from build123d import *

# Parameters (mm, degrees)
F0_R     = 11.05
F1_DEPTH = 3.5
F2_DEPTH = 2.5


with BuildPart() as f1:
    # F0 (on Top) → F1 (new body, symmetric)
    with BuildSketch(Plane.XY):
        with BuildLine():
            Line((16.4067340595, 45.3467654298), (8.4209065052, 43.9228967168))
            ThreePointArc((8.4209065052, 43.9228967168), (15.6672457553, 43.3028857057), (21.6327540042, 39.1427706216))
            Line((21.6327540042, 39.1427706216), (16.4067340595, 45.3467654298))
        make_face()
        with BuildLine():
            Line((0.4350802259, 42.4990282311), (-2.3247269809, 34.8711645999))
            ThreePointArc((-2.3247269809, 34.8711645999), (1.8353876304, 40.8366725376), (8.4209065052, 43.9228967168))
            Line((8.4209065052, 43.9228967168), (0.4350802259, 42.4990282311))
        make_face()
        with BuildLine():
            ThreePointArc((24.9371199001, 30.0910388701), (24.7259953173, 27.6645131258), (24.0989665638, 25.3109125396))
            Line((24.0989665638, 25.3109125396), (26.8587737337, 32.9387760688))
            Line((26.8587737337, 32.9387760688), (21.6327540042, 39.1427706216))
            ThreePointArc((21.6327540042, 39.1427706216), (24.0852004265, 34.9090436873), (24.9371199001, 30.0910388701))
        make_face()
        with BuildLine():
            Line((-5.0845339335, 27.2433016714), (-0.112226606, 21.3404981668))
            Line((-0.112226606, 21.3404981668), (-0.1100221461, 21.3465910994))
            ThreePointArc((-0.1100221461, 21.3465910994), (-2.9782076587, 27.8205341493), (-2.3247269809, 34.8711645999))
            Line((-2.3247269809, 34.8711645999), (-5.0845339335, 27.2433016714))
        make_face()
        with BuildLine():
            Line((13.7432325819, 16.334399733), (13.741028122, 16.3283068004))
            Line((13.741028122, 16.3283068004), (21.3391595743, 17.6830495091))
            Line((21.3391595743, 17.6830495091), (24.0989665638, 25.3109125396))
            ThreePointArc((24.0989665638, 25.3109125396), (20.0897974955, 19.474390384), (13.7432325819, 16.334399733))
        make_face()
        with BuildLine():
            Line((-0.112226606, 21.3404981668), (0.1414857049, 21.0393072268))
            ThreePointArc((0.1414857049, 21.0393072268), (0.0146461468, 21.1920605869), (-0.1100221461, 21.3465910994))
            Line((-0.1100221461, 21.3465910994), (-0.112226606, 21.3404981668))
        make_face()
        with BuildLine():
            ThreePointArc((13.7432325819, 16.334399733), (13.5485483413, 16.2954128005), (13.3533326046, 16.2591809003))
            Line((13.3533326046, 16.2591809003), (13.741028122, 16.3283068004))
            Line((13.741028122, 16.3283068004), (13.7432325819, 16.334399733))
        make_face()
        Polygon((18.5375268448, -10.5730579916), (11.3795390219, -11.8493233304), (10.9594646934, -13.0103717128), (9.743930135, -13.227100864), (7.2702144289, -20.064232828), (4.6443903041, -27.3217790413), (15.0964299783, -39.7297684023), (31.0680838119, -36.8820312036), (36.5876979713, -21.6263046439), (26.1356582971, -9.2183152829), align=None)
        with Locations((20.6160441377, -24.4740418426)):
            Circle(F0_R, mode=Mode.SUBTRACT)
        Polygon((-16.7470447626, -2.98598898), (-16.3269704341, -1.8249405976), (-21.0112425509, 3.7359260276), (-25.9835498784, 9.6387295322), (-41.955203712, 6.7909923335), (-47.4748178714, -8.4647342262), (-37.0227781972, -20.8727235872), (-21.0511243636, -18.0249863885), (-18.4253002388, -10.7674401752), (-15.9515845328, -3.9303082112), align=None)
        with Locations((-31.5031640378, -5.6169970275)):
            Circle(F0_R, mode=Mode.SUBTRACT)
        with BuildLine():
            ThreePointArc((0.1414857049, 21.0393072268), (2.850394978, 18.5665626335), (6.106993819, 16.8791921162))
            ThreePointArc((6.106993819, 16.8791921162), (9.6893501995, 16.092187212), (13.3533326046, 16.2591809003))
            ThreePointArc((13.3533326046, 16.2591809003), (13.5485483413, 16.2954128005), (13.7432325819, 16.334399733))
            ThreePointArc((13.7432325819, 16.334399733), (20.0897974955, 19.474390384), (24.0989665638, 25.3109125396))
            ThreePointArc((24.0989665638, 25.3109125396), (24.7259953173, 27.6645131258), (24.9371199001, 30.0910388701))
            ThreePointArc((24.9371199001, 30.0910388701), (24.0852004265, 34.9090436873), (21.6327540042, 39.1427706216))
            ThreePointArc((21.6327540042, 39.1427706216), (15.6672457553, 43.3028857057), (8.4209065052, 43.9228967168))
            ThreePointArc((8.4209065052, 43.9228967168), (1.8353876304, 40.8366725376), (-2.3247269809, 34.8711645999))
            ThreePointArc((-2.3247269809, 34.8711645999), (-2.9782076587, 27.8205341493), (-0.1100221461, 21.3465910994))
            ThreePointArc((-0.1100221461, 21.3465910994), (0.0146461468, 21.1920605869), (0.1414857049, 21.0393072268))
        make_face()
        with BuildLine():
            ThreePointArc((21.9371199001, 30.0910388701), (17.2337915702, 21.0454731767), (7.1276613096, 19.7002270103))
            ThreePointArc((7.1276613096, 19.7002270103), (4.5404482301, 39.1366045634), (21.9371199001, 30.0910388701))
        make_face(mode=Mode.SUBTRACT)
        Polygon((6.5830402991, 15.0520414616), (5.3675057407, 14.8353123104), (4.5720455108, 15.7796315416), (-2.5859423121, 14.5033662028), (-10.9594646934, 13.0103717128), (-13.853254728, 5.0121913664), (-16.3269704341, -1.8249405976), (-15.5315102042, -2.7692598288), (-15.9515845328, -3.9303082112), (-11.2673124159, -9.4911748364), (-5.7875800692, -15.9963606927), (2.5859423121, -14.5033662028), (9.743930135, -13.227100864), (10.1640044635, -12.0660524816), (11.3795390219, -11.8493233304), (13.853254728, -5.0121913664), (16.7470447626, 2.98598898), (11.2673124159, 9.4911748364), align=None)
        with BuildLine():
            ThreePointArc((3.7594585905, 10.3908118598), (9.0455656933, 6.3466716701), (11.05, 0))
            ThreePointArc((11.05, 0), (-9.0455656933, -6.3466716701), (3.7594585905, 10.3908118598))
        make_face(mode=Mode.SUBTRACT)
        with BuildLine():
            Line((6.106993819, 16.8791921162), (5.7875800692, 15.9963606927))
            Line((5.7875800692, 15.9963606927), (6.5830402991, 15.0520414616))
            Line((6.5830402991, 15.0520414616), (13.3533326046, 16.2591809003))
            ThreePointArc((13.3533326046, 16.2591809003), (9.6893501995, 16.092187212), (6.106993819, 16.8791921162))
        make_face()
        with BuildLine():
            Line((4.5720455108, 15.7796315416), (5.7875800692, 15.9963606927))
            Line((5.7875800692, 15.9963606927), (6.106993819, 16.8791921162))
            ThreePointArc((6.106993819, 16.8791921162), (2.850394978, 18.5665626335), (0.1414857049, 21.0393072268))
            Line((0.1414857049, 21.0393072268), (4.5720455108, 15.7796315416))
        make_face()
        Polygon((4.5720455108, 15.7796315416), (5.3675057407, 14.8353123104), (5.7875800692, 15.9963606927), align=None)
        Polygon((5.7875800692, 15.9963606927), (5.3675057407, 14.8353123104), (6.5830402991, 15.0520414616), align=None)
        Polygon((10.9594646934, -13.0103717128), (11.3795390219, -11.8493233304), (10.1640044635, -12.0660524816), (9.743930135, -13.227100864), align=None)
        Polygon((-15.5315102042, -2.7692598288), (-16.3269704341, -1.8249405976), (-16.7470447626, -2.98598898), (-15.9515845328, -3.9303082112), align=None)
    extrude(amount=F1_DEPTH, both=True)

    # F0 (on Top) → F2 (join, symmetric)
    with BuildSketch(Plane.XY):
        Polygon((-2.5859423121, 14.5033662028), (4.5720455108, 15.7796315416), (0.1414857049, 21.0393072268), (-0.112226606, 21.3404981668), align=None)
        Polygon((13.3533326046, 16.2591809003), (6.5830402991, 15.0520414616), (11.2673124159, 9.4911748364), (13.741028122, 16.3283068004), align=None)
        Polygon((18.5375268448, -10.5730579916), (13.853254728, -5.0121913664), (11.3795390219, -11.8493233304), align=None)
        Polygon((7.2702144289, -20.064232828), (9.743930135, -13.227100864), (2.5859423121, -14.5033662028), align=None)
        Polygon((-11.2673124159, -9.4911748364), (-15.9515845328, -3.9303082112), (-18.4253002388, -10.7674401752), align=None)
        Polygon((-16.3269704341, -1.8249405976), (-13.853254728, 5.0121913664), (-21.0112425509, 3.7359260276), align=None)
    extrude(amount=F2_DEPTH, both=True)


solid = f1.part
For this review, take the finished solid that the model builds, in its own axes (mm). A direction names the side the tool comes from. Give positions to 0.01 mm unless a question says otherwise; leave off trailing zeros. Loops run counter-clockwise (first coordinate to the right, second up) from the corner with the lowest first, then second, coordinate; pieces in that order, holes last.
Item 1: For line 1 along X through (y, z) = (-13, -0.5); line 2 along X through (y, z) = (40, 0.5); line 3 along Y through (x, z) = (-30.5, -2.25), list the stretches that pass through material, from the lowest coordinate up.
Item 2: Tool access review of faces 4 (the flat face through (-15, -8, 2.5)), 5 (the flat face through (4.895, -17.245, -0.035)), 6 (the flat face through (7, -16, -2.5)): name each direction out of +Z, -Z, +X, -X, +Y, -Y from which nothing blocks a thin tool from reaching the whole face with its end or side.
Item 3: Take a section at A-A, the plane x = 28. State the section outline as (y, z) points.
Item 4: Insertion check: pin 1 (5.5 mm diameter, centred on x = 4.5, y = -17.5, fed in from +Z); pin 2 (7.5 mm diameter, centred on x = -14.5, y = -8, fed in from +Z); pin 3 (2 mm diameter, centred on x = -14.5, y = -8, fed in from -Z); pin 4 (4 mm diameter, centred on x = -13.5, z = -2, fed in from -Y). Each pin has a flat end and moves straight along its axis. Give the tip position at first contact, or say it passes through.
Item 5: Take a section at C-C, the plane z = 1.5. Give the number of separate pieces and of enclosed holes in the cut face, and give its area (3 significant figures).
Item 6: Take a section at B-B, the plane y = 0. State the section outline as (x, z) points.
Item 7: Draft analysis for pull direction Y (two halves, no side actions). For faces 1 (the flat face through (-17, 2, -2.5)), 2 (the flat face through (-33.858, 8.235, 0.049)), 3 (the flat face through (-1.33, 17.97, -0.04)), state which applies: +Y half, -Y half, draft (parallel to the pull), parting line (faces both ways), or undercut.
Calculated:
1. line 1: x = -43.65 to -39.72, -23.28 to -19.23, -8.31 to 29.32
1. line 2: x = -0.47 to 6, 15.78 to 20.91
1. line 3: y = -19.71 to -16.62, 5.39 to 8.83
2. face 4: +Z, -Y
2. face 5: +Z, -Z
2. face 6: -Z
3. outline: (-37.43, -3.5) - (-32.69, -3.5) - (-32.69, 3.5) - (-37.43, 3.5) - close; (-16.25, -3.5) - (-11.43, -3.5) - (-11.43, 3.5) - (-16.25, 3.5) - close
4. pin 1: stops at z = 2.5
4. pin 2: stops at z = 3.5
4. pin 3: stops at z = -2.5
4. pin 4: stops at y = -10.25
5. separate pieces: 1
5. enclosed holes: 4
5. area: 1,400 mm2
6. outline: (-44.41, -3.5) - (-41.02, -3.5) - (-41.02, 3.5) - (-44.41, 3.5) - close; (-21.99, -3.5) - (-17.86, -3.5) - (-17.86, -2.5) - (-15.67, -2.5) - (-15.67, -3.5) - (-11.05, -3.5) - (-11.05, 3.5) - (-15.67, 3.5) - (-15.67, 2.5) - (-17.86, 2.5) - (-17.86, 3.5) - (-21.99, 3.5) - close; (11.05, -3.5) - (15.67, -3.5) - (15.67, 3.5) - (11.05, 3.5) - close
7. face 1: draft
7. face 2: +Y half
7. face 3: undercut
